Design review of the part built by this model. Coordinates are the model's own, in mm. Coordinates: 2 decimals unless noted, no trailing zeros. Write each loop counter-clockwise with the first axis right and the second up, starting at its lowest first coordinate (ties: lowest second). Pieces come first, ordered by that corner, then holes.
Q1. For probe 1 along X at (y, z) = (0, 6); probe 2 along Y at (x, z) = (-10, 1.5); probe 3 along X at (y, z) = (1.5, 6.5), list the stretches that pass through material, from the lowest coordinate up.
Q2. Take a section at A-A (x = 10). Give the boundary of the cut face in (y, z), and give its area (3 significant figures).
Q3. Take a section at C-C (y = 0). Give the boundary of the cut face in (x, z).
Q4. Insertion check: pin 1 (5.5 mm diameter, centred on x = -10, y = 0, fed in from +Z). The pin has a flat end and moves straight along its axis. Give the tip position at first contact, or say it passes through.
Q5. Take a section at B-B (z = 6.75). Give the boundary of the cut face in (x, y), and give its area (3 significant figures).
Autodesk Inventor part; units mm, degrees
ref_plane "YZ Plane" through (0, 0, 0) normal (1, 0, 0) x (0, 1, 0)
ref_plane "XZ Plane" through (0, 0, 0) normal (0, 1, 0) x (-1, 0, 0)
ref_plane "XY Plane" through (0, 0, 0) normal (0, 0, 1) x (1, 0, 0)
sketch "スケッチ1" plane through (0, 0, 0) normal (0, 0, 1) x (1, 0, 0)
  line L0 (15, -5) -> (-15, -5)
  line L1 (-15, -5) -> (-15, 5)
  line L2 (-15, 5) -> (15, 5)
  line L3 (15, 5) -> (15, -5)
  line L4 (15, -5) -> (-15, 5) construction
  line L5 (-15, -5) -> (15, 5) construction
  line L6 (-15, 0) -> (15, 0)
  circle A0 centre (-10, 0) radius 1.75
  circle A1 centre (10, 0) radius 1.75
  point P0 (0, 0)
  point P1 (0, 0)
  dimension "d0" = 30
  dimension "d1" = 10
  dimension "d2" = 3.5
  dimension "d3" = 3.5
  dimension "d4" = 20
  dimension "d5" = 10
extrude "押し出し1" add sketch "スケッチ1" along normal blind 8 contours L0 L1 L6 A0 A1 L3 | L6 A1 A0 L1 L2 L3
fillet "フィレット1" radius 2 4 edges at (-15, 5, 4) (15, 5, 4) (15, -5, 4) (-15, -5, 4)
properties part number "gear_enco_plate"
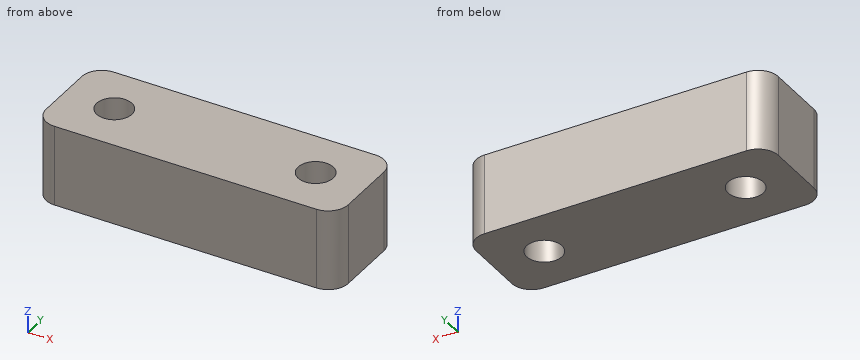
Response:
1. probe 1: x = -15 to -11.75, -8.25 to 8.25, 11.75 to 15
1. probe 2: y = -5 to -1.75, 1.75 to 5
1. probe 3: x = -15 to -10.9, -9.1 to 9.1, 10.9 to 15
2. outline: (-5, 0) - (-1.75, 0) - (-1.75, 8) - (-5, 8) - close; (1.75, 0) - (5, 0) - (5, 8) - (1.75, 8) - close
2. area: 52.0 mm2
3. outline: (-15, 0) - (-11.75, 0) - (-11.75, 8) - (-15, 8) - close; (-8.25, 0) - (8.25, 0) - (8.25, 8) - (-8.25, 8) - close; (11.75, 0) - (15, 0) - (15, 8) - (11.75, 8) - close
4. pin 1: stops at z = 8
5. outline: (-15, -3) arc R2 ccw to (-13, -5) - (13, -5) arc R2 ccw to (15, -3) - (15, 3) arc R2 ccw to (13, 5) - (-13, 5) arc R2 ccw to (-15, 3) - close; hole circle Ø3.5 at (-10, 0); hole circle Ø3.5 at (10, 0)
5. area: 277 mm2
